Autodesk Inventor part; units mm, degrees
ref_plane "YZ Plane" through (0, 0, 0) normal (1, 0, 0) x (0, 1, 0)
ref_plane "XZ Plane" through (0, 0, 0) normal (0, 1, 0) x (-1, 0, 0)
ref_plane "XY Plane" through (0, 0, 0) normal (0, 0, 1) x (1, 0, 0)
ref_plane "Plano de trabajo1" through (0, 27, 0) normal (0, 1, 0) x (1, 0, 0)
sketch "Boceto2" plane through (0, 27, 0) normal (0, 1, 0) x (1, 0, 0)
  line L0 (0, 10) -> (0, 15)
  line L1 (0, 15) -> (11.8906, 15)
  line L2 (0, 10) -> (0, 5)
  line L3 (0, 5) -> (15.0689, 5)
  line L4 (0, 5) -> (7, 5)
  line L5 (7, 5) -> (7, 15)
  line L6 (6.4875, 15) -> (4.4875, 15)
  circle A0 centre (4.4875, 15) radius 1.5
  circle A1 centre (4.4875, 5) radius 1.5
  line L7 (-42, 6) -> (-42, 0)
  line L8 (0, 0) -> (-42, 0)
  line L9 (-42, 0) -> (0, 0)
  line L10 (-21, 0) -> (-21, 36.5425)
  circle A2 centre (-46.4875, 15) radius 1.5
  circle A3 centre (-46.4875, 5) radius 1.5
  line L11 (0, 0) -> (1, 0)
  line L12 (1, 0) -> (8, 0)
  line L13 (8, 0) -> (8, 20)
  line L14 (8, 20) -> (1, 20)
  line L15 (1, 20) -> (1, 0)
  line L16 (-42, 10) -> (-42, 15)
  line L17 (-42, 15) -> (-53.8906, 15)
  line L18 (-42, 10) -> (-42, 5)
  line L19 (-42, 5) -> (-49, 5)
  line L20 (-49, 5) -> (-49, 15)
  line L21 (-48.4875, 15) -> (-46.4875, 15)
  circle A4 centre (-46.4875, 15) radius 1.5
  circle A5 centre (-46.4875, 5) radius 1.5
  line L22 (-42, 0) -> (-43, 0)
  line L23 (-43, 0) -> (-50, 0)
  line L24 (-50, 0) -> (-50, 20)
  line L25 (-50, 20) -> (-43, 20)
  line L26 (-43, 20) -> (-43, 0)
  line L27 (-43, 20) -> (-43, 21)
  line L28 (-43, 21) -> (1, 21)
  line L29 (1, 21) -> (1, 20)
  line L30 (-43, 0) -> (-43, -1)
  line L31 (-43, -1) -> (1, -1)
  line L32 (1, -1) -> (1, 0)
  line L33 (-50, 20) -> (-50, 24)
  line L34 (-50, 24) -> (8, 24)
  line L35 (-50, 0) -> (-50, -4)
  line L36 (-50, -4) -> (8, -4)
  line L37 (8, -4) -> (8, 0)
  line L38 (8, 24) -> (8, 19.2948)
  line L39 (-42, 10) -> (-42, 7)
  line L40 (-42, 7) -> (-58.0956, 7)
  line L41 (-51, 14) -> (-51, 6)
  line L42 (-42, 10) -> (-42, 13)
  line L43 (-42, 13) -> (-56.402, 13)
  point P0 (0, 20)
  point P1 (-42, 20)
  point P2 (-50, 13)
  point P3 (-43, 13)
  point P4 (-43, 7)
  point P5 (-50, 7)
  dimension "d8" = 5
  dimension "d9" = 5
  dimension "d10" = 7
  dimension "d11" = 2
  dimension "d12" = 3
  dimension "d13" = 3
  dimension "d14" = 1
  dimension "d15" = 7
  dimension "d16" = 1
  dimension "d17" = 1
  dimension "d18" = 4
  dimension "d19" = 4
  dimension "d22" = 3
  dimension "d23" = 3
extrude "Extrusión2" add sketch "Boceto2" along normal blind 4 contours L15 L14 L13 L1 A0 | L1 A0 L5 L3 A1 L15 | L3 A1 L13 L12 L15 | L29 L28 L10 L34 L38 L14 | L12 L37 L36 L35 L23 L30 L31 L32 | L28 L27 L25 L33 L34 L10 | L5 L1 L13 L3 | L23 L24 L40 L20 L19 A3 L26 | L26 L17 A2 L24 L25 | L19 A3 L20 L40 L26 | L26 L43 L20 L17 A2 | L17 L20 L43 L24
sketch "Boceto3" plane through (8, 27, -24) normal (0, 0, -1) x (-1, 0, 0)
  point P0 (8, -27)
sketch "Boceto4" plane through (8, 27, -24) normal (0, 0, -1) x (-1, 0, 0)
  line L0 (0, 4) -> (58, 4)
  line L1 (58, 4) -> (58, 18.1)
  line L2 (58, 18.1) -> (0, 18.1)
  line L3 (0, 18.1) -> (0, 4)
  line L4 (58, 18.1) -> (58, 22.1)
  line L5 (58, 18.1) -> (58, 32.1)
  line L6 (58, 32.1) -> (0, 32.1)
  line L7 (0, 32.1) -> (0, 18.1)
  line L8 (58, 18.1) -> (58, 28.6)
  line L9 (58, 28.6) -> (36.9156, 28.6)
  line L10 (8, -6.3468) -> (8, 18.1)
  line L11 (8, 18.1) -> (18.1, 18.1)
  line L12 (18.1, 18.1) -> (41.1, 18.1)
  line L13 (41.1, 18.1) -> (51.1, 18.1)
  line L14 (51.1, 18.1) -> (51.1, 26.6579)
  line L15 (51.1, 26.6579) -> (51.1, 31.1823)
  line L16 (51.1, 18.1) -> (51.1, 18)
  line L17 (51.1, 18.1) -> (51.2, 18.1)
  line L18 (51.2, 18.1) -> (51.2, 31.1)
  line L19 (51.2, 31.1) -> (41.1, 31.1)
  line L20 (41.1, 31.1) -> (41.1, 18.1)
  line L21 (51.2, 28.6) -> (49.2, 28.6)
  line L22 (41.1, 28.6) -> (43.1, 28.6)
  line L23 (43.1, 28.6) -> (43.15, 28.6)
  circle A0 centre (43.15, 28.6) radius 1.5
  line L24 (43.15, 28.6) -> (49.15, 28.6)
  circle A1 centre (49.15, 28.6) radius 1.5
  point P0 (8, -27)
  point P1 (8, 4)
  dimension "d24" = 14.1
  dimension "d25" = 4
  dimension "d26" = 14
  dimension "d27" = 10.5
  dimension "d28" = 10.1
  dimension "d29" = 23
  dimension "d30" = 10
  dimension "d31" = 0.1
  dimension "d32" = 0.1
  dimension "d33" = 13
  dimension "d34" = 10.1
  dimension "d35" = 2
  dimension "d36" = 2
  dimension "d38" = 0.05
  dimension "d39" = 3
  dimension "d40" = 6
  dimension "d41" = 3
extrude "Extrusión3" add sketch "Boceto4" along normal blind 5 contours L3 L2 L10 L0 | L10 L2 L1 L0 | L7 L6 L5 L9 L18 L19 L20 L2 | L2 L18 L9 L5 L4
sketch "Boceto5" plane through (8, 27, -29) normal (0, 0, -1) x (-1, 0, 0)
  line L0 (51.2, 18.1) -> (41.1, 18.1)
  line L1 (51.2, 18.1) -> (51.2, 28.6)
  line L2 (51.2, 31.1) -> (51.2, 18.1)
  line L3 (51.2, 28.6) -> (49.15, 28.6)
  circle A0 centre (49.15, 28.6) radius 1.5
  line L4 (49.15, 28.6) -> (43.15, 28.6)
  circle A1 centre (43.15, 28.6) radius 1.5
  line L5 (41.1, 18.1) -> (51.2, 18.1)
  line L6 (51.2, 18.1) -> (51.2, 31.1)
  line L7 (51.2, 31.1) -> (41.1, 31.1)
  line L8 (41.1, 31.1) -> (41.1, 18.1)
  point P0 (8, -27)
  dimension "d44" = 10.5
  dimension "d45" = 2.05
  dimension "d46" = 3
  dimension "d47" = 6
  dimension "d48" = 3
extrude "Extrusión4" add sketch "Boceto5" against normal blind 3
sketch "Boceto6" plane through (-50, 31, -24) normal (0, -1, 0) x (1, 0, 0)
  line L0 (58, -5) -> (0, -5)
  line L1 (0, 0) -> (58, 0)
  line L2 (58, 0) -> (58, -5)
  line L3 (58, -5) -> (0, -5)
  line L4 (0, -5) -> (0, 0)
  point P0 (50, 24)
extrude "Extrusión5" add sketch "Boceto6" along normal blind 4
properties part number "servo pinza"
Build history of the part. All positions in model axes, mm. A direction names the side the tool comes from. Coordinates: 2 decimals unless noted, no trailing zeros. Order: outer loops, then holes, each group sorted by start corner. A loop starts at its lowest first (then second) coordinate and runs counter-clockwise, first axis right, second up. Notation, with made-up numbers: (5.5, 40.25) -> (36.5, 40.25) arc R16 cw to (36.5, 61.25) -> close; hole circle Ø9 at (-19, -26.5). An arc over 180 degrees is marked (long way). Answer in a Markdown table with one row per item. Add a question column.
Q1. Which spindle directions (+Z, -Z, +X, -X, +Y, -Y) get a long thin tool onto all of the face, cutting with end or side? Do faces 1 (the face through (-43, 29, -17)), 2 (the face through (-38, 45.1, -25)), 3 (the face through (-21, 45, -24)), 4 (the face through (-35.956, 56.865, -27.521)). Say none if no direction does.
Q2. Band-saw the part on A-A, the plane z = -18. List the corners of the cut face in (x, y).
Q3. Band-saw the part on B-B, the plane x = -2.5. List the corners of the cut face in (y, z).
Q4. Band-saw the part on C-C, the plane x = -41.15. List the corners of the cut face in (y, z).
Q5. Mould opens along X. For faces 5 (the face through (-38, 58.1, -25)), 6 (the face through (3.38, 28.97, -3.99)), 7 (the face through (-46, 29, -13)), 8 (the face through (-50, 40, -25)) say: +X half, -X half, draft (parallel to the pull), parting line (faces both ways), or undercut.
Q6. Drop flat-ended pins along their axis: pin 1 (1 mm diameter, centred on y = 33, z = 0.5, fed in from +X); pin 2 (5 mm diameter, centred on x = -46.49, z = -15, fed in from +Y); pin 3 (3.5 mm diameter, centred on x = -41.15, y = 55.6, fed in from +Z). Give the stop position or say it passes through.
Q7. Wall check: line 1 along X through (y, z) = (29.95, -15); line 2 along Y through (x, z) = (-4.5, -23); line 3 along Z through (x, y) = (1.5, 40.5). Give the ranges that are in metal, low to high. Write a range as [from, to].
Q8. Band-saw the part on D-D, the plane y = 34. List the corners of the cut face in (x, z).
Answers follow:
| question | item | result |
|---|---|---|
| 1 | face 1 | +Y, -Y |
| 1 | face 2 | +Z |
| 1 | face 3 | +Z, +X, -X, +Y |
| 1 | face 4 | +Z, -Z |
| 2 | outline | (-50, 27) -> (-43, 27) -> (-43, 31) -> (-50, 31) -> close; (1, 27) -> (8, 27) -> (8, 31) -> (1, 31) -> close |
| 3 | outline | (27, -29) -> (59.1, -29) -> (59.1, -24) -> (31, -24) -> (31, -21) -> (27, -21) -> close; (27, 1) -> (31, 1) -> (31, 4) -> (27, 4) -> close |
| 4 | outline | (27, -29) -> (54.1, -29) -> (54.1, -26) -> (45.1, -26) -> (45.1, -24) -> (31, -24) -> (31, -21) -> (27, -21) -> close; (27, 1) -> (31, 1) -> (31, 4) -> (27, 4) -> close; (57.1, -29) -> (59.1, -29) -> (59.1, -24) -> (58.1, -24) -> (58.1, -26) -> (57.1, -26) -> close |
| 5 | face 5 | undercut |
| 5 | face 6 | undercut |
| 5 | face 7 | draft |
| 5 | face 8 | -X half |
| 6 | pin 1 | through |
| 6 | pin 2 | y = 31 |
| 6 | pin 3 | z = -26 |
| 7 | line 1 | [-50, -47.99], [-44.99, -43], [1, 2.99], [5.99, 8] |
| 7 | line 2 | [27, 31] |
| 7 | line 3 | [-29, -24] |
| 8 | outline | (-50, -29) -> (8, -29) -> (8, -24) -> (-50, -24) -> close |
